from build123d import *

# Parameters (mm, degrees)
BOSS_EXTRUDE1_DEPTH = 30
SKETCH3_R           = 3
CUT_EXTRUDE2_DEPTH  = 504.388517946


with BuildPart() as part:
    # Sketch1 → Boss-Extrude1 (new body)
    with BuildSketch(Plane.XY):
        Polygon((500, 50), (463.602976573, -50), (-500, -50), (-500, 50), align=None)
    extrude(amount=BOSS_EXTRUDE1_DEPTH)

    # Sketch3 → Cut-Extrude2 (cut, through all)
    with BuildSketch(Plane.XY.offset(30)):
        with Locations((110, 0)):
            Circle(SKETCH3_R)
        with Locations((280, 0)):
            Circle(SKETCH3_R)
    extrude(amount=-CUT_EXTRUDE2_DEPTH, mode=Mode.SUBTRACT)


solid = part.part
Can you work these out from the model? Positions are in its coordinate system, mm. Round coordinates to 2 decimals unless told otherwise and drop trailing zeros. Loops run counter-clockwise (first coordinate to the right, second up) from the corner with the lowest first, then second, coordinate; pieces in that order, holes last. Notation, with made-up numbers: (31, -10) - (36, -10) arc R9 ccw to (36, 5) - close; hole circle Ø10 at (-25, 36.25). An arc over 180 degrees is marked (long way). Answer in a Markdown table with one row per item. Add a question column.
Q1. I want a section at A-A on z = 13.75. List the corners of the cut face in (x, y) for me, and give its area (3 significant figures).
Q2. I want a section at B-B on y = -13. List the corners of the cut face in (x, z) for me.
Q3. I need wall thicknesses on L1, parallel to Y at x = 110, z = 11; L2, parallel to X at y = 4, z = 3.25; L3, parallel to X at y = 13.5, z = 9.75. Which ranges of each line are inside material? Lowest first, please.
Q4. For pin 1 Ø4 at (y, z) = (-1.5, 9) entering from +X; pin 2 Ø4 at (y, z) = (7, 25.5) entering from +X, each with a flat end and sliding along its axis, tell me the tip position at first contact or that it passes through.
A:
| question | item | result |
|---|---|---|
| 1 | outline | (-500, -50) - (463.6, -50) - (500, 50) - (-500, 50) - close; hole circle Ø6 at (110, 0); hole circle Ø6 at (280, 0) |
| 1 | area | 98,100 mm^2 |
| 2 | outline | (-500, 0) - (477.07, 0) - (477.07, 30) - (-500, 30) - close |
| 3 | L1 | -50 to -3, 3 to 50 |
| 3 | L2 | -500 to 483.26 |
| 3 | L3 | -500 to 486.72 |
| 4 | pin 1 | x = 481.98 |
| 4 | pin 2 | x = 485.08 |
